from build123d import *

# Parameters (mm, degrees)
SALIENTE_EXTRUIR1_START      = 0.1
SALIENTE_EXTRUIR1_DEPTH      = 1.3
SALIENTE_EXTRUIR3_START      = 0.1
SALIENTE_EXTRUIR3_DEPTH      = 1.3
SALIENTE_EXTRUIR3_DEPTH_BACK = 6.5
SALIENTE_EXTRUIR2_START      = 1.4
CROQUIS1_3_W                 = 45.8
CROQUIS1_3_H                 = 27.5
CROQUIS1_3_R                 = 1.65
SALIENTE_EXTRUIR2_DEPTH      = 5.5
REDONDEO2_R                  = 2


with BuildPart() as part:
    # Croquis1 → Saliente-Extruir1 (new body)
    with BuildSketch(Plane.XY.offset(SALIENTE_EXTRUIR1_START)):
        with BuildLine():
            Line((-13.85, -3.2), (-59.65, -3.2))
            Line((-59.65, -3.2), (-59.65, -9.05))
            Line((-59.65, -9.05), (-47.282475165, -9.05))
            ThreePointArc((-47.282475165, -9.05), (-46.803420224, -6.334895379), (-44.5, -7.85))
            ThreePointArc((-44.5, -7.85), (-44.634895379, -8.503420224), (-45.017524835, -9.05))
            Line((-45.017524835, -9.05), (-27.282475165, -9.05))
            ThreePointArc((-27.282475165, -9.05), (-26.803420224, -6.334895379), (-24.5, -7.85))
            ThreePointArc((-24.5, -7.85), (-24.634895379, -8.503420224), (-25.017524835, -9.05))
            Line((-25.017524835, -9.05), (-13.85, -9.05))
            Line((-13.85, -9.05), (-13.85, -3.2))
        make_face()
    extrude(amount=SALIENTE_EXTRUIR1_DEPTH)



with BuildPart() as body_2:
    # Croquis1<5> → Saliente-Extruir3 (new, two sides)
    with BuildSketch(Plane.XY.offset(SALIENTE_EXTRUIR3_START)) as saliente_extruir3_sk:
        with BuildLine():
            Line((-47.282489505, -21.65), (-59.65, -21.65))
            Line((-59.65, -21.65), (-59.65, -30.7))
            Line((-59.65, -30.7), (-13.85, -30.7))
            Line((-13.85, -30.7), (-13.85, -21.65))
            Line((-13.85, -21.65), (-25.017510495, -21.65))
            ThreePointArc((-25.017510495, -21.65), (-24.634891475, -22.196575296), (-24.5, -22.849986467))
            ThreePointArc((-24.5, -22.849986467), (-26.803411171, -24.365094992), (-27.282489505, -21.65))
            Line((-27.282489505, -21.65), (-45.017510495, -21.65))
            ThreePointArc((-45.017510495, -21.65), (-44.634891475, -22.196575296), (-44.5, -22.849986467))
            ThreePointArc((-44.5, -22.849986467), (-46.803411171, -24.365094992), (-47.282489505, -21.65))
        make_face()
    extrude(amount=SALIENTE_EXTRUIR3_DEPTH)
    extrude(saliente_extruir3_sk.sketch, amount=-SALIENTE_EXTRUIR3_DEPTH_BACK)


with BuildPart() as part_1:
    add(part.part)

    add(body_2.part)  # Saliente-Extruir2 merges body 2
    # Croquis1<3> → Saliente-Extruir2 (add)
    with BuildSketch(Plane.XY.offset(SALIENTE_EXTRUIR2_START)):
        with Locations((-36.75, -16.95)):
            Rectangle(CROQUIS1_3_W, CROQUIS1_3_H)
        with Locations(Location((-46.15, -22.849986467, 0), (0, 0, 133.342442907))):
            Circle(CROQUIS1_3_R, mode=Mode.SUBTRACT)
        with Locations(Location((-26.15, -22.849986467, 0), (0, 0, 133.342442907))):
            Circle(CROQUIS1_3_R, mode=Mode.SUBTRACT)
        with Locations(Location((-26.15, -7.85, 0), (0, 0, 226.658241773))):
            Circle(CROQUIS1_3_R, mode=Mode.SUBTRACT)
        with Locations(Location((-46.15, -7.85, 0), (0, 0, 226.658241773))):
            Circle(CROQUIS1_3_R, mode=Mode.SUBTRACT)
        with Locations((-54.65, -15.35)):
            Circle(CROQUIS1_3_R, mode=Mode.SUBTRACT)
        with Locations((-29.65, -15.35)):
            Circle(CROQUIS1_3_R, mode=Mode.SUBTRACT)
    extrude(amount=SALIENTE_EXTRUIR2_DEPTH)

    # Redondeo2
    redondeo2_edges = [part_1.edges().sort_by_distance(p)[0] for p in [
        (-59.65, -16.95, 6.9),
    ]]
    fillet(redondeo2_edges, radius=REDONDEO2_R)


solid = part_1.part
Can you work these out from the model? Positions are in its coordinate system, mm. A direction names the side the tool comes from. Round coordinates to 2 decimals unless told otherwise and drop trailing zeros. Write each loop counter-clockwise with the first axis right and the second up, starting at its lowest first coordinate (ties: lowest second). Pieces come first, ordered by that corner, then holes. Notation, with made-up numbers: (-13.5, 84) -> (28.5, 84) arc R30 cw to (28.5, 111) -> close; hole circle Ø9 at (88, 70.25). An arc over 180 degrees is marked (long way). Use one line per item in the form item = value. Start each with the question number.
Q1. Imagine slicing it at D-D (y = -5.25). Please give me the cut outline in (x, z).
Q2. Imagine slicing it at B-B (x = -26.15). Please give me the cut outline in (y, z), then the cut area to 3 significant figures.
Q3. Which directions (+Z, -Z, +X, -X, +Y, -Y) give clear straight access to the entire face, cutting with the end or side of a thin tool? Please do faces 5 (the face through (-36, -17, 6.9)), 6 (the face through (-37, -6, 0.1)), 7 (the face through (-37, -15, 1.4)).
Q4. I'm going to push flat-ended pins straight in: P1, Ø4.5, axis at x = -26.15, y = -7.85, coming from the +Z side; P2, Ø12, axis at x = -19.5, y = -13, coming from the -Z side; P3, Ø6.5, axis at x = -42, y = -16, coming from the -Z side; P4, Ø2.5, axis at x = -36, z = -1.5, coming from the +Y side. Where does each tip first touch, or does it pass through?
Q5. We'd pull the mould along Y, two halves only. Please class faces 1 (the face through (-28.126, -15.982, 4.111)), 2 (the face through (-37, -30.7, 0)), 3 (the face through (-37, -3.2, 3)), 4 (the face through (-37, -26, -6.4)): +Y half, -Y half, draft (parallel to the pull), parting line (faces both ways), or undercut.
Q6. Imagine slicing it at C-C (x = -54.65). Please give me the cut outline in (y, z), then the cut area to 3 significant figures.
Q7. If I drill on probe 1 along Y at (x, z) = (-26.15, 4.6); probe 2 along X at (y, z) = (-7.85, 4.25); probe 3 along Y at (x, z) = (-26, 1.25), over which ranges is the centre line in solid material (lowest first)? Write a range as [from, to].
Q8. Imagine slicing it at A-A (y = -15.35). Please give me the cut outline in (x, z).
Worked out:
q1.outline = (-59.65, 0.1) -> (-13.85, 0.1) -> (-13.85, 6.9) -> (-57.65, 6.9) arc R2 ccw to (-59.65, 4.9) -> close
q2.outline = (-30.7, -6.4) -> (-24.5, -6.4) -> (-24.5, 6.9) -> (-30.7, 6.9) -> close; (-21.2, 1.4) -> (-9.5, 1.4) -> (-9.5, 6.9) -> (-21.2, 6.9) -> close; (-6.2, 0.1) -> (-3.2, 0.1) -> (-3.2, 6.9) -> (-6.2, 6.9) -> close
q2.area = 167 mm^2
q3.face_5 = +Z, +X, -X, +Y, -Y
q3.face_6 = -Z, +X, -X, +Y
q3.face_7 = -Z, +X, -X
q4.P1 = 6.9
q4.P2 = 0.1
q4.P3 = 1.4
q4.P4 = -21.65
q5.face_1 = undercut
q5.face_2 = -Y half
q5.face_3 = +Y half
q5.face_4 = draft
q6.outline = (-30.7, -6.4) -> (-21.65, -6.4) -> (-21.65, 1.4) -> (-17, 1.4) -> (-17, 6.9) -> (-30.7, 6.9) -> close; (-13.7, 1.4) -> (-9.05, 1.4) -> (-9.05, 0.1) -> (-3.2, 0.1) -> (-3.2, 6.9) -> (-13.7, 6.9) -> close
q6.area = 211 mm^2
q7.probe_1 = [-30.7, -24.5], [-21.2, -9.5], [-6.2, -3.2]
q7.probe_2 = [-59.65, -47.8], [-44.5, -27.8], [-24.5, -13.85]
q7.probe_3 = [-30.7, -24.49], [-6.21, -3.2]
q8.outline = (-59.65, 1.4) -> (-56.3, 1.4) -> (-56.3, 6.9) -> (-57.65, 6.9) arc R2 ccw to (-59.65, 4.9) -> close; (-53, 1.4) -> (-31.3, 1.4) -> (-31.3, 6.9) -> (-53, 6.9) -> close; (-28, 1.4) -> (-13.85, 1.4) -> (-13.85, 6.9) -> (-28, 6.9) -> close
